```python
from build123d import *

# Parameters (mm, degrees)
BOSS_EXTRUDE1_DEPTH = 22
CUT_EXTRUDE1_DEPTH  = 12
CHAMFER1_SIZE       = 18
FILLET1_R           = 5
FILLET2_R           = 5


with BuildPart() as part:
    # Sketch2 → Boss-Extrude1 (new body)
    with BuildSketch(Plane.XY):
        with BuildLine():
            Line((14.99994, 31.165268255), (24.99994, 31.165268255))
            Line((24.99994, 31.165268255), (24.99994, 9.365268255))
            Line((24.99994, 9.365268255), (14.99994, 9.365268255))
            Line((14.99994, 9.365268255), (12.999948, 9.365268255))
            Line((12.999948, 9.365268255), (4.5, 9.365268255))
            ThreePointArc((4.5, 9.365268255), (4.005025253, 9.160243002), (3.8, 8.665268255))
            Line((3.8, 8.665268255), (3.8, 7.407802905))
            ThreePointArc((3.8, 7.407802905), (4.005025253, 6.912828158), (4.5, 6.707802905))
            Line((4.5, 6.707802905), (7.736453928, 6.707802905))
            ThreePointArc((7.736453928, 6.707802905), (7.957266257, 6.624965773), (8.049967, 6.408109491))
            Line((8.049967, 6.408109491), (8.049967, 4.425516287))
            ThreePointArc((8.049967, 4.425516287), (8.027131012, 4.310712023), (7.96209962, 4.213385667))
            Line((7.96209962, 4.213385667), (4.036581333, 0.28786738))
            ThreePointArc((4.036581333, 0.28786738), (3.939254977, 0.222835988), (3.824450713, 0.2))
            Line((3.824450713, 0.2), (-3.824450713, 0.2))
            ThreePointArc((-3.824450713, 0.2), (-3.939254977, 0.222835988), (-4.036581333, 0.28786738))
            Line((-4.036581333, 0.28786738), (-7.96209962, 4.213385667))
            ThreePointArc((-7.96209962, 4.213385667), (-8.027131012, 4.310712023), (-8.049967, 4.425516287))
            Line((-8.049967, 4.425516287), (-8.049967, 6.408109491))
            ThreePointArc((-8.049967, 6.408109491), (-7.957266257, 6.624965773), (-7.736453928, 6.707802905))
            Line((-7.736453928, 6.707802905), (-4.5, 6.707802905))
            ThreePointArc((-4.5, 6.707802905), (-4.005025253, 6.912828158), (-3.8, 7.407802905))
            Line((-3.8, 7.407802905), (-3.8, 8.665268255))
            ThreePointArc((-3.8, 8.665268255), (-4.005025253, 9.160243002), (-4.5, 9.365268255))
            Line((-4.5, 9.365268255), (-12.999948, 9.365268255))
            Line((-12.999948, 9.365268255), (-14.99994, 9.365268255))
            Line((-14.99994, 9.365268255), (-14.99994, 31.165268255))
            Line((-14.99994, 31.165268255), (14.99994, 31.165268255))
        make_face()
    extrude(amount=BOSS_EXTRUDE1_DEPTH)

    # Sketch3 → Cut-Extrude1 (cut)
    with BuildSketch(Plane(origin=(24.99994, 0, 0), x_dir=(0, 0, -1), z_dir=(1, 0, 0))):
        with BuildLine():
            Line((-17.45, 31.165268255), (-4.55, 31.165268255))
            Line((-4.55, 31.165268255), (-4.55, 27.615268255))
            Line((-4.55, 27.615268255), (-4.85, 23.109490465))
            ThreePointArc((-4.85, 23.109490465), (-11, 14.715268255), (-17.15, 23.109490465))
            Line((-17.15, 23.109490465), (-17.45, 27.615268255))
            Line((-17.45, 27.615268255), (-17.45, 31.165268255))
        make_face()
    extrude(amount=-CUT_EXTRUDE1_DEPTH, mode=Mode.SUBTRACT)

    # Chamfer1
    chamfer1_edges = [part.edges().sort_by_distance(p)[0] for p in [
        (-14.99994, 31.165268255, 11),
    ]]
    chamfer(chamfer1_edges, length=CHAMFER1_SIZE)

    # Fillet1
    fillet1_edges = [part.edges().sort_by_distance(p)[0] for p in [
        (-14.99994, 13.165268255, 11),
        (3.00006, 31.165268255, 11),
    ]]
    fillet(fillet1_edges, radius=FILLET1_R)

    # Fillet2
    fillet2_edges = [part.edges().sort_by_distance(p)[0] for p in [
        (24.99994, 31.165268255, 2.275),
        (24.99994, 31.165268255, 19.725),
    ]]
    fillet(fillet2_edges, radius=FILLET2_R)

    # Cut-Sweep7: sweep along a path in Sketch43
    with BuildLine(Plane.XY.offset(22)) as cut_sweep7_path:
        Line((-14.99994, 9.365268255), (-4.8, 9.365268255))
        ThreePointArc((-4.8, 9.365268255), (-4.092893219, 9.072375036), (-3.8, 8.365268255))
        Line((-3.8, 8.365268255), (-3.8, 7.707802905))
        ThreePointArc((-3.8, 7.707802905), (-4.092893219, 7.000696124), (-4.8, 6.707802905))
        Line((-4.8, 6.707802905), (-7.049967, 6.707802905))
        ThreePointArc((-7.049967, 6.707802905), (-7.757073781, 6.414909686), (-8.049967, 5.707802905))
        Line((-8.049967, 5.707802905), (-8.049967, 4.715466609))
        ThreePointArc((-8.049967, 4.715466609), (-7.973846533, 4.332783177), (-7.757073781, 4.008359828))
        Line((-7.757073781, 4.008359828), (-4.241607172, 0.492893219))
        ThreePointArc((-4.241607172, 0.492893219), (-3.917183823, 0.276120467), (-3.534500391, 0.2))
        Line((-3.534500391, 0.2), (3.534500391, 0.2))
        ThreePointArc((3.534500391, 0.2), (3.917183823, 0.276120467), (4.241607172, 0.492893219))
        Line((4.241607172, 0.492893219), (7.757073781, 4.008359828))
        ThreePointArc((7.757073781, 4.008359828), (7.973846533, 4.332783177), (8.049967, 4.715466609))
        Line((8.049967, 4.715466609), (8.049967, 5.707802905))
        ThreePointArc((8.049967, 5.707802905), (7.757073781, 6.414909686), (7.049967, 6.707802905))
        Line((7.049967, 6.707802905), (4.8, 6.707802905))
        ThreePointArc((4.8, 6.707802905), (4.092893219, 7.000696124), (3.8, 7.707802905))
        Line((3.8, 7.707802905), (3.8, 8.365268255))
        ThreePointArc((3.8, 8.365268255), (4.092893219, 9.072375036), (4.8, 9.365268255))
        Line((4.8, 9.365268255), (14.99994, 9.365268255))
        Line((14.99994, 9.365268255), (24.99994, 9.365268255))
    # Sketch4 → Cut-Sweep7 (sweep, cut)
    with BuildSketch(Plane.ZY.offset(14.99994)):
        Polygon((22, 10.072375036), (22.707106781, 9.365268255), (22, 8.658161474), (20.776291928, 8.963134662), (21.292893219, 9.365268255), align=None)
    cut_sweep7 = sweep(path=cut_sweep7_path.line, mode=Mode.SUBTRACT)

    # Mirror1: Cut-Sweep7 across plane
    add(cut_sweep7.mirror(Plane(origin=(0, 0, 11), x_dir=(1, 0, 0), z_dir=(0, 0, -1))), mode=Mode.SUBTRACT)


solid = part.part
```
Geometry check sheet. Reference: the model listing, model coordinates, mm. A direction names the side the tool comes from. Coordinates: 2 decimals unless noted, no trailing zeros. Order: outer loops, then holes, each group sorted by start corner. A loop starts at its lowest first (then second) coordinate and runs counter-clockwise, first axis right, second up. Notation, with made-up numbers: M 61,15.25 L 90,15.25 A4 ccw 90,21.25 Z; hole C -19.5,42 d8. An arc over 180 degrees is marked long. One line per question, with ' | ' between items. Start each with the question number.
Item 1: Cross-section at D-D on x = 20.5. Enter the section's corners in (y, z), then the cut area to 3 significant figures.
Item 2: Cross-section at C-C on y = 17. Enter the section's corners in (x, z), then the cut area to 3 significant figures.
Item 3: Draft check along Y on faces 4 (the flat face through (6.03, 2.28, 10.86)), 5 (the flat face through (-6.105, 22.06, 10.846)), 6 (the conical face through (7.847, 6.487, 0.855)). Enter one of: pulls with the +Y half, pulls with the -Y half, needs draft (parallel to the pull), parting line crosses it, or undercut.
Item 4: Cross-section at B-B on x = 6.5. Enter the section's corners in (y, z), then the cut area to 3 significant figures.
Item 5: Gauge pin test, flat ends, axial feed: pin 1 (11.5 mm diameter, centred on y = 21.17, z = 11, fed in from +X); pin 2 (2 mm diameter, centred on y = 5, z = 18.5, fed in from -X); pin 3 (1 mm diameter, centred on y = 8, z = 13, fed in from -X). Record the tip position at first contact, or that the pin passes through.
Item 6: Material ranges on L1, parallel to X at y = 5.5, z = 17.5; L2, parallel to Y at x = 22, z = 11.25; L3, parallel to Y at x = 7, z = 19.25, recorded low to high. Write a range as [from, to].
Item 7: Set-up check for faces 1 (the conical face through (3.89, 9.25, 0.44)), 2 (the conical face through (3.912, 6.8, 21.563)), 3 (the flat face through (-6, 6.708, 11)): record each of +Z, -Z, +X, -X, +Y, -Y from which the full face is reachable in a straight line by a thin tool's end or side.
Findings:
1) outline: M 9.37,0.71 L 10.07,0 L 31.14,0 L 31.14,4.55 L 27.62,4.55 L 23.11,4.85 A6.45 cw long 23.11,17.15 L 27.62,17.45 L 31.14,17.45 L 31.14,22 L 10.07,22 L 9.37,21.29 Z | area: 286 mm²
2) outline: M -11.17,0 L 25,0 L 25,6.08 L 13,6.08 L 13,15.92 L 25,15.92 L 25,22 L -11.17,22 Z | area: 677 mm²
3) face 4: pulls with the -Y half | face 5: pulls with the +Y half | face 6: undercut
4) outline: M 2.75,0.71 L 3.75,0 L 6,0 L 6.71,0.71 L 6.71,21.29 L 6,22 L 3.75,22 L 2.75,21.29 Z; M 9.37,0.71 L 10.07,0 L 31.17,0 L 31.17,22 L 10.07,22 L 9.37,21.29 Z | area: 565 mm²
5) pin 1: stops at x = 13 | pin 2: stops at x = -8.05 | pin 3: stops at x = -3.8
6) L1: x = [-8.05, 8.05] | L2: y = [9.37, 14.72] | L3: y = [3.25, 6.71], [9.37, 31.17]
7) face 1: -Z, +X | face 2: +Z, +X | face 3: +Z, -Z, -X
